Check sheet for the modelled part. Datum: model origin and axes. Units: mm. Coordinates: 2 decimals unless noted, no trailing zeros. Loops run counter-clockwise (first coordinate to the right, second up) from the corner with the lowest first, then second, coordinate; pieces in that order, holes last.
```python
from build123d import *

# Parameters (mm, degrees)
SKETCH1_W                                      = 85.999999704
SKETCH1_H                                      = 84.074
BOSS_EXTRUDE1_DEPTH                            = 4.999999906
CSK_FOR_4_FLAT_HEAD_MACHINE_SCREW1_D           = 3.2639
CSK_FOR_4_FLAT_HEAD_MACHINE_SCREW1_CSINK_D     = 5.715
CSK_FOR_4_FLAT_HEAD_MACHINE_SCREW1_CSINK_ANGLE = 82


with BuildPart() as part:
    # Sketch1 → Boss-Extrude1 (new body)
    with BuildSketch(Plane.XY):
        Rectangle(SKETCH1_W, SKETCH1_H)
    extrude(amount=BOSS_EXTRUDE1_DEPTH)

    # CSK for #4 Flat Head Machine Screw1 (through all)
    with Locations(Plane.XY.offset(4.999999906)):
        with Locations((-39.189999852, 38.227), (39.189999852, 38.227), (-39.189999852, -38.227), (39.189999852, -38.227)):
            CounterSinkHole(CSK_FOR_4_FLAT_HEAD_MACHINE_SCREW1_D / 2, CSK_FOR_4_FLAT_HEAD_MACHINE_SCREW1_CSINK_D / 2, counter_sink_angle=CSK_FOR_4_FLAT_HEAD_MACHINE_SCREW1_CSINK_ANGLE)


solid = part.part
```
1) Mould release check, pull along Y, two halves, no side actions. Record for faces 1 (the flat face through (-1, 1, 5)), 2 (the flat face through (-1, 42.037, 2)), 3 (the cylindrical face through (-37.987, 39.33, 1.77)): +Y half, -Y half, draft (parallel to the pull), parting line (faces both ways), or undercut.
Answer sheet:
face 1: draft
face 2: +Y half
face 3: undercut
2) Scan lines: line 1 (Y direction, x = -39.19, z = 1.1); line 2 (Y direction, x = 39, z = 3.55). Record each from-to range of solid material in increasing order.
Answer sheet:
line 1: y = -42.04 to -39.86, -36.6 to 36.6, 39.86 to 42.04
line 2: y = -42.04 to -39.85, -36.61 to 36.61, 39.85 to 42.04
3) Section check A-A on x = -39.19. Enter the section's corners in (y, z).
Answer sheet:
outline: (-42.04, 0) - (-39.86, 0) - (-39.86, 3.59) - (-41.08, 5) - (-42.04, 5) - close; (-36.6, 0) - (36.6, 0) - (36.6, 3.59) - (35.37, 5) - (-35.37, 5) - (-36.6, 3.59) - close; (39.86, 0) - (42.04, 0) - (42.04, 5) - (41.08, 5) - (39.86, 3.59) - close
